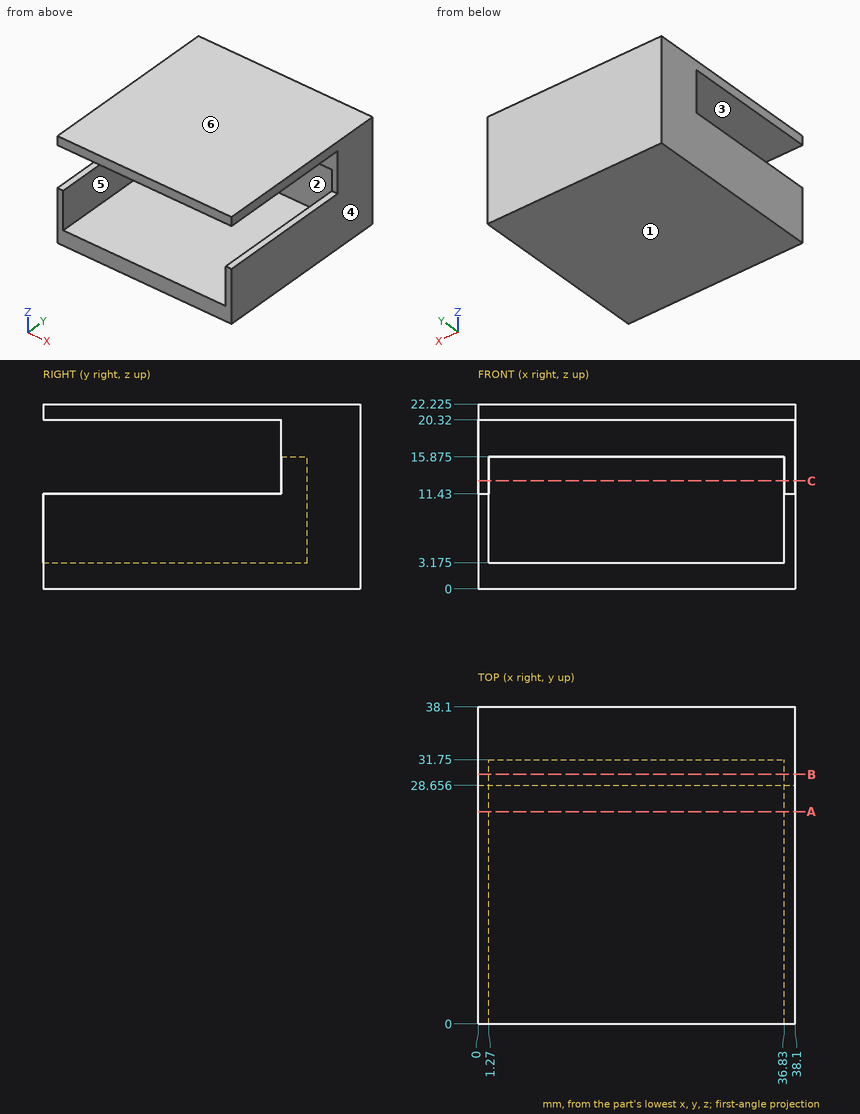
Input: dimensioned drawing with shaded views. Units: mm. Origin: part minimum x, y, z. A direction names the side the tool comes from. Coordinates: 2 decimals unless noted, no trailing zeros. Loops run counter-clockwise (first coordinate to the right, second up) from the corner with the lowest first, then second, coordinate; pieces in that order, holes last. Notation, with made-up numbers: M 3,-36 L 41,-36 A32 cw 41,-4 Z; hole C -5,65.5 d2. An arc over 180 degrees is marked long. One line per item, written item: value.
(1) Pin query (flat end, axial travel): pin 1 (1.5 mm diameter, centred on x = 24.5, y = 29.5, fed in from -Z); pin 2 (7 mm diameter, centred on x = 22.5, z = 15.5, fed in from -Y); pin 3 (4 mm diameter, centred on x = 14.5, z = 9, fed in from -Y). Return the tip coordinate at first contact, or that it passes through.
Filled in:
pin 1: z = 0
pin 2: y = 28.66
pin 3: y = 31.75
(2) Section A-A (y = 25.5). Output: boundary loops of the cut face in (x, z) (1 decimal).
Filled in:
outline: M 0,0 L 38.1,0 L 38.1,11.4 L 36.8,11.4 L 36.8,3.2 L 1.3,3.2 L 1.3,11.4 L 0,11.4 Z; M 0,20.3 L 38.1,20.3 L 38.1,22.2 L 0,22.2 Z
(3) Section C-C (z = 13). Output: boundary loops of the cut face in (x, y), and give its area (3 significant figures).
Filled in:
outline: M 0,28.66 L 1.27,28.66 L 1.27,31.75 L 36.83,31.75 L 36.83,28.66 L 38.1,28.66 L 38.1,38.1 L 0,38.1 Z
area: 250 mm^2
(4) Reachability of the marked faces 1, 2 and 3 from +Z, -Z, +X, -X, +Y, -Y: full face, straight path, thin tool, end or side. Return the list, or none.
Filled in:
face 1: -Z, +X, -X, +Y, -Y
face 2: -Y
face 3: +X, -X, -Y
(5) Section B-B (y = 30). Output: boundary loops of the cut face in (x, z) (1 decimal).
Filled in:
outline: M 0,0 L 38.1,0 L 38.1,22.2 L 0,22.2 Z; hole M 1.3,3.2 L 36.8,3.2 L 36.8,15.9 L 1.3,15.9 Z
(6) Line query: line 1 along Z through (x, y) = (21, 13) (1 decimal); line 2 along X through (y, z) = (28, 6.5); line 3 along Z through (x, y) = (15, 30) (1 decimal). Output: solid intervals per line, ascending. Write a range as from..to.
Filled in:
line 1: 0..3.2, 20.3..22.2
line 2: 0..1.27, 36.83..38.1
line 3: 0..3.2, 15.9..22.2
(7) Pull-direction query (X, two-part tool) for the marked faces 4, 5 and 6; classes: +X half, -X half, draft (parallel to the pull), parting line (faces both ways), or undercut.
Filled in:
face 4: +X half
face 5: undercut
face 6: draft
